Geometry check sheet. Reference: drawing and pictorial views, mm from the part's lowest x, y, z. A direction names the side the tool comes from. Coordinates: 2 decimals unless noted, no trailing zeros. Loops run counter-clockwise (first coordinate to the right, second up) from the corner with the lowest first, then second, coordinate; pieces in that order, holes last. Notation, with made-up numbers: (-38, 59.25) -> (5, 59.25) arc R17 ccw to (5, 64.25) -> close; hole circle Ø9 at (24, -12.5). An arc over 180 degrees is marked (long way). Answer as a JSON object with one key per item and string values.
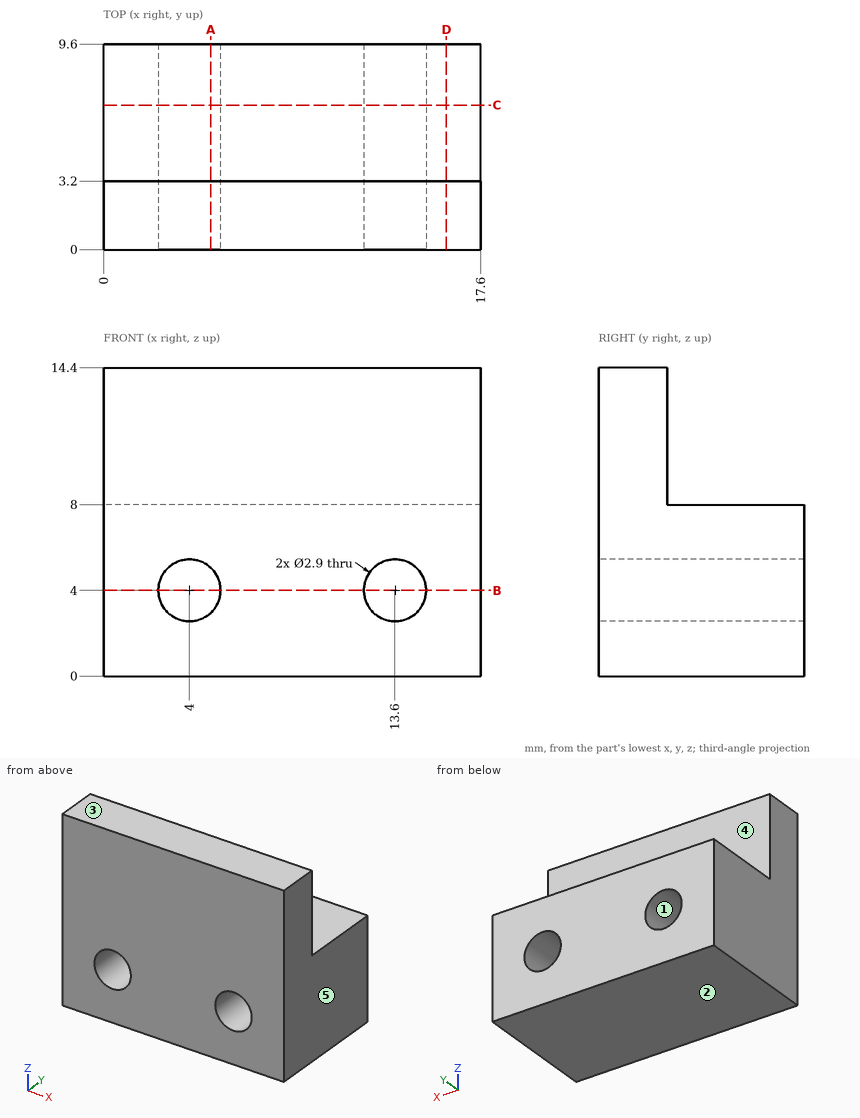
1. Section check A-A, the plane x = 5. Record the boundary of the cut face in (y, z).
Evaluation:
{"outline": "(0, 0) -> (9.6, 0) -> (9.6, 2.95) -> (0, 2.95) -> close; (0, 5.05) -> (9.6, 5.05) -> (9.6, 8) -> (3.2, 8) -> (3.2, 14.4) -> (0, 14.4) -> close"}
2. Thickness scan on probe 1 along X at (y, z) = (7, 4); probe 2 along Y at (x, z) = (15.25, 8.25); probe 3 along Z at (x, y) = (4, 2.25). Record the ranges inside material, lowest first. Write a range as from..to.
Evaluation:
{"probe 1": "x = 0..2.55, 5.45..12.15, 15.05..17.6", "probe 2": "y = 0..3.2", "probe 3": "z = 0..2.55, 5.45..14.4"}
3. Section check D-D, the plane x = 16. Record the boundary of the cut face in (y, z).
Evaluation:
{"outline": "(0, 0) -> (9.6, 0) -> (9.6, 8) -> (3.2, 8) -> (3.2, 14.4) -> (0, 14.4) -> close"}
4. Depth check by flat-ended pin: P1, Ø4, axis at x = 5.5, y = 7.5, coming from the +Z side; P2, Ø1, axis at y = 4, z = 10, coming from the -X side; P3, Ø1.9, axis at x = 9.5, z = 11, coming from the +Y side. Enter the tip coordinate at first touch or a pass-through.
Evaluation:
{"P1": "stops at z = 8", "P2": "passes through", "P3": "stops at y = 3.2"}
5. Section check B-B, the plane z = 4. Record the boundary of the cut face in (x, y), then the cut area to 3 significant figures.
Evaluation:
{"outline": "(0, 0) -> (2.55, 0) -> (2.55, 9.6) -> (0, 9.6) -> close; (5.45, 0) -> (12.15, 0) -> (12.15, 9.6) -> (5.45, 9.6) -> close; (15.05, 0) -> (17.6, 0) -> (17.6, 9.6) -> (15.05, 9.6) -> close", "area": "113 mm^2"}
6. Section check C-C, the plane y = 6.75. Record the boundary of the cut face in (x, z), then the cut area to 3 significant figures.
Evaluation:
{"outline": "(0, 0) -> (17.6, 0) -> (17.6, 8) -> (0, 8) -> close; hole circle Ø2.9 at (4, 4); hole circle Ø2.9 at (13.6, 4)", "area": "128 mm^2"}
7. Tool access check on the marked faces 4 and 5. Record the directions out of +Z, -Z, +X, -X, +Y, -Y that give a thin tool (end or side, any length) a straight path to the whole face; none if there is none.
Evaluation:
{"face 4": "+Z, +X, -X, +Y", "face 5": "+Z, -Z, +X, +Y, -Y"}
8. Mould release check, pull along Z, two halves, no side actions. Record for the marked faces 1, 2 and 3: released by +Z, released by -Z, zero draft, split by the parting line, or undercut.
Evaluation:
{"face 1": "undercut", "face 2": "released by -Z", "face 3": "released by +Z"}
